Input: dimensioned drawing with shaded views. Units: mm. Origin: part minimum x, y, z. A direction names the side the tool comes from. Give positions to 0.01 mm unless a question says otherwise; leave off trailing zeros. Loops run counter-clockwise (first coordinate to the right, second up) from the corner with the lowest first, then second, coordinate; pieces in that order, holes last. Notation, with made-up numbers: M -26,36 L 24,36 A27 ccw 24,71 Z; hole C 18,-8.75 d9. An arc over 180 degrees is marked long. Use CSV: the item, a comma, the result in double quotes. Start each with the question number.
Q1. Section A-A, the plane x = 19. Output: boundary loops of the cut face in (y, z), plus the area to 3 significant figures.
Q2. Section D-D, the plane z = 37. Output: boundary loops of the cut face in (x, y).
Q3. Reachability of the marked faces 1 and 2 from +Z, -Z, +X, -X, +Y, -Y: full face, straight path, thin tool, end or side. Return the list, or none.
Q4. Pin query (flat end, axial travel): pin 1 (12 mm diameter, centred on x = 27, z = 31.5, fed in from +Y); pin 2 (2 mm diameter, centred on x = 31, y = 52, fed in from +Z); pin 3 (3 mm diameter, centred on x = 22, z = 40.5, fed in from -Y); pin 4 (1.5 mm diameter, centred on x = 16, y = 18.5, fed in from -Z). Return the tip coordinate at first contact, or that it passes through.
Q5. Section B-B, the plane y = 20. Output: boundary loops of the cut face in (x, z).
Q6. Section C-C, the plane y = 77. Output: boundary loops of the cut face in (x, z), plus the area to 3 significant figures.
Q7. Material intervals for line 1 along Y through (x, z) = (19, 3.9); line 2 along Z through (x, y) = (33, 106); line 3 along Y through (x, z) = (12.5, 31), sorted ascending.
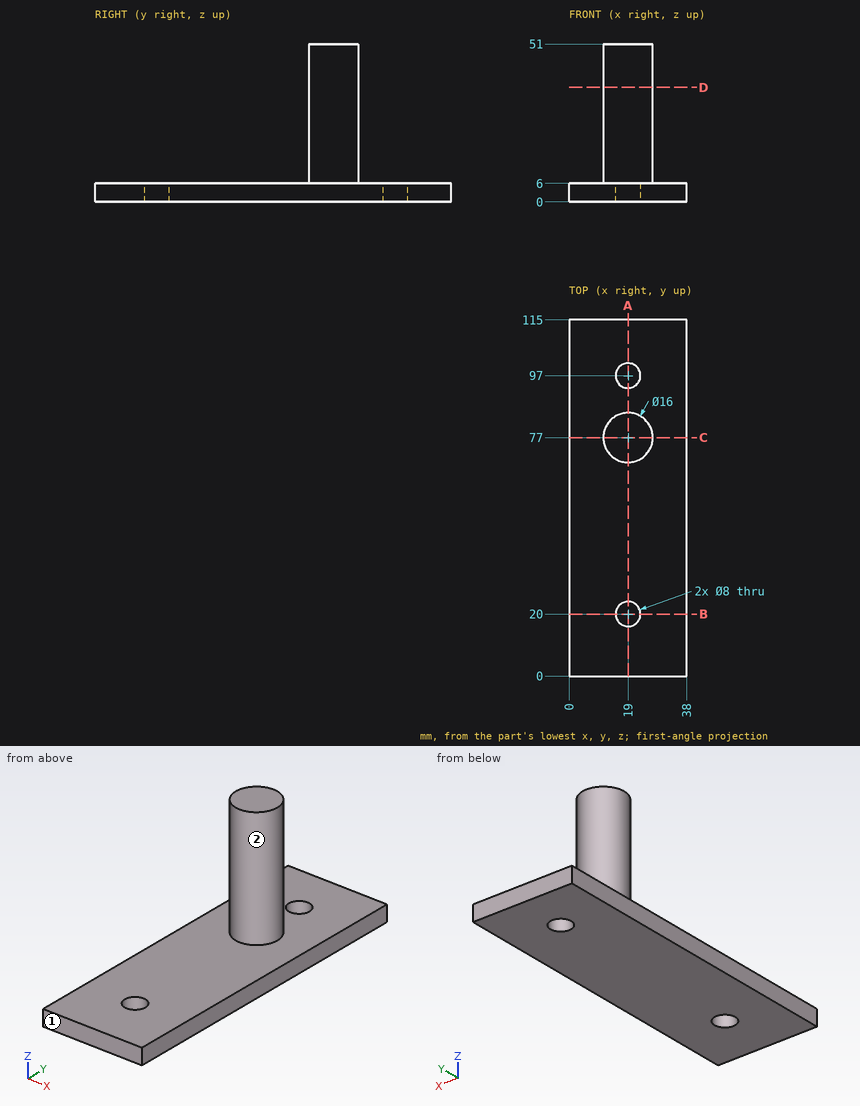
A:
1,outline,"M 0,0 L 16,0 L 16,6 L 0,6 Z; M 24,0 L 93,0 L 93,6 L 85,6 L 85,51 L 69,51 L 69,6 L 24,6 Z; M 101,0 L 115,0 L 115,6 L 101,6 Z"
1,area,"1,310 mm^2"
2,outline,"C 19,77 d16"
3,face 1,"+Z, -Z, +X, -X, -Y"
3,face 2,"+Z"
4,pin 1,"y = 84.75"
4,pin 2,"z = 6"
4,pin 3,"y = 69.14"
4,pin 4,"z = 0"
5,outline,"M 0,0 L 15,0 L 15,6 L 0,6 Z; M 23,0 L 38,0 L 38,6 L 23,6 Z"
6,outline,"M 0,0 L 38,0 L 38,6 L 27,6 L 27,51 L 11,51 L 11,6 L 0,6 Z"
6,area,"948 mm^2"
7,line 1,"0 to 16, 24 to 93, 101 to 115"
7,line 2,"0 to 6"
7,line 3,"72.34 to 81.66"
